Design review of the part built by this model. Coordinates are the model's own, in mm. A direction names the side the tool comes from. Give positions to 0.01 mm unless a question says otherwise; leave off trailing zeros. Loops run counter-clockwise (first coordinate to the right, second up) from the corner with the lowest first, then second, coordinate; pieces in that order, holes last. Notation, with made-up numbers: (7.25, 76.25) -> (46.25, 76.25) arc R19 cw to (46.25, 88.25) -> close; hole circle Ø10 at (39, 56.5). An arc over 180 degrees is marked (long way). Use CSV: the item, a comma, the result in double quotes. Start each with the question number.
Item 1: We need section B-B (y = 3.75). State the section outline as (x, z) points, plus the area to 3 significant figures.
Item 2: For faces 4 (the face through (-0.59, 4.46, 0.3)), 5 (the face through (2, -3, 0.6)), 6 (the face through (0, 0, 0.5)), list the 3-axis set-ups (+Z, -Z, +X, -X, +Y, -Y) from which the entire face can be reached by the end or side of a thin tool; tool diameter is ignored.
Item 3: The part is to be moulded in two halves that separate along Y. For faces 1 (the face through (-1.1, 1.1, 0)), 2 (the face through (-2.539, -1.947, 3.262)), 3 (the face through (-0.17, 1.29, 0.25)), say which applies: +Y half, -Y half, draft (parallel to the pull), parting line (faces both ways), or undercut.
Item 4: Wall thickness on line 1 along Y through (x, z) = (0, 0.4); line 2 along Z through (x, y) = (3.5, 1.5); line 3 along Z through (x, y) = (0.25, 1.75): over which ranges is each line inside the solid? List them lowest first. Write a range as from..to.
Item 5: We need section A-A (z = 1). State the section outline as (x, y) points, plus the area to 3 significant figures.
Item 6: Clearance check with flat-ended pins moving along their axes: pin 1 (1 mm diameter, centred on x = 3, y = -1, fed in from +Z); pin 2 (3 mm diameter, centred on x = 2.5, y = 2, fed in from +Z); pin 3 (3 mm diameter, centred on x = 0, z = 2.5, fed in from -Y); pin 4 (2 mm diameter, centred on x = 1, y = -0.5, fed in from -Z). State where each tip first meets the part, or that it passes through.
from build123d import *

# Parameters (mm, degrees)
F0_R     = 4.5
F0_R_2   = 3.2
F0_R_3   = 1.3
F1_DEPTH = 0.6
F2_DEPTH = 8
F3_R     = 2
F4_DEPTH = 0.5


with BuildPart() as f1:
    # F0 (on Top) → F1 (new body)
    with BuildSketch(Plane.XY):
        Circle(F0_R)
        Circle(F0_R_2, mode=Mode.SUBTRACT)
        Circle(F0_R_2)
        Circle(F0_R_3, mode=Mode.SUBTRACT)
    extrude(amount=F1_DEPTH)

    # F0 (on Top) → F2 (join)
    with BuildSketch(Plane.XY):
        Circle(F0_R_2)
        Circle(F0_R_3, mode=Mode.SUBTRACT)
        Circle(F0_R_3)
    extrude(amount=F2_DEPTH)

    # F3
    f3_edges = [f1.edges().sort_by_distance(p)[0] for p in [
        (-3.2, 0, 8),
    ]]
    fillet(f3_edges, radius=F3_R)

    # F0 (on Top) → F4 (cut)
    with BuildSketch(Plane.XY):
        Circle(F0_R_3)
    extrude(amount=F4_DEPTH, mode=Mode.SUBTRACT)


solid = f1.part
Results found:
1,outline,"(-2.49, 0) -> (2.49, 0) -> (2.49, 0.6) -> (-2.49, 0.6) -> close"
1,area,"2.98 mm²"
2,face 4,"+Z, -Z"
2,face 5,"+Z"
2,face 6,"-Z"
3,face 1,"draft"
3,face 2,"parting line"
3,face 3,"undercut"
4,line 1,"-4.5..-1.3, 1.3..4.5"
4,line 2,"0..0.6"
4,line 3,"0..7.92"
5,outline,"circle Ø6.4 at (0, 0)"
5,area,"32.2 mm²"
6,pin 1,"z = 7.36"
6,pin 2,"z = 7.94"
6,pin 3,"y = -3.2"
6,pin 4,"z = 0"
